Check sheet for the modelled part. Datum: model origin and axes. Units: mm. Round coordinates to 2 decimals unless told otherwise and drop trailing zeros. Loops run counter-clockwise (first coordinate to the right, second up) from the corner with the lowest first, then second, coordinate; pieces in that order, holes last. Notation, with made-up numbers: (43, 71.5) -> (95, 71.5) arc R23 ccw to (95, 81.5) -> close; hole circle Ø3 at (-6.75, 19.5). An arc over 180 degrees is marked (long way). One line per question, with ' | ' between items.
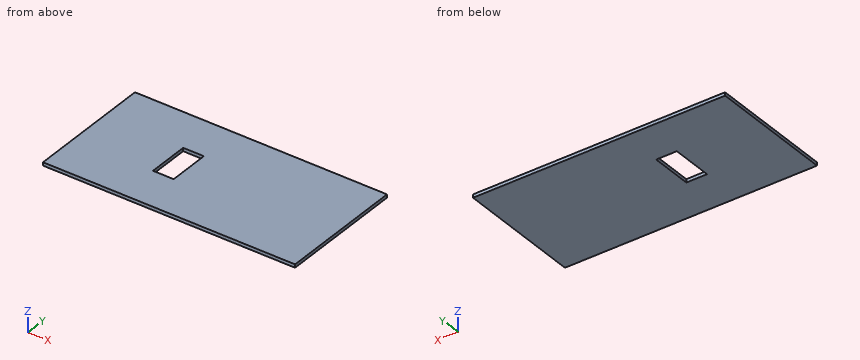
Autodesk Inventor part; units mm, degrees
ref_plane "YZ Plane" through (0, 0, 0) normal (1, 0, 0) x (0, 1, 0)
ref_plane "XZ Plane" through (0, 0, 0) normal (0, 1, 0) x (-1, 0, 0)
ref_plane "XY Plane" through (0, 0, 0) normal (0, 0, 1) x (1, 0, 0)
sketch "Sketch1" plane through (0, 0, 0) normal (0, 0, 1) x (1, 0, 0)
  line L0 (0, 0) -> (1219.2, 0)
  line L1 (1219.2, 0) -> (1219.2, 609.6)
  line L2 (1219.2, 609.6) -> (0, 609.6)
  line L3 (0, 609.6) -> (0, 0)
  dimension "d0" = 1219.2
  dimension "d1" = 609.6
extrude "Extrusion1" add sketch "Sketch1" along normal blind 15.875
sketch "Sketch6" plane through (0, 0, 15.875) normal (0, 0, 1) x (1, 0, 0)
  line L0 (482.6, 404.8) -> (382.6, 404.8)
  line L1 (482.6, 204.8) -> (382.6, 204.8)
  line L2 (382.6, 204.8) -> (382.6, 404.8)
  line L3 (482.6, 404.8) -> (482.6, 204.8)
extrude "Extrusion5" cut sketch "Sketch6" against normal blind 90
properties part number "Window Gyp Board"
(1) Sectioned sample at B-B, the plane z = 7.5. Record the cut outline in (x, y).
Answer:
outline: (0, 0) -> (1219.2, 0) -> (1219.2, 609.6) -> (0, 609.6) -> close; hole (382.6, 204.8) -> (482.6, 204.8) -> (482.6, 404.8) -> (382.6, 404.8) -> close
(2) Scan lines: probe 1 along X at (y, z) = (241, 3); probe 2 along Y at (x, z) = (442, 2). Record each from-to range of solid material in increasing order.
Answer:
probe 1: x = 0 to 382.6, 482.6 to 1219.2 | probe 2: y = 0 to 204.8, 404.8 to 609.6
(3) Sectioned sample at A-A, the plane y = 229. Record the cut outline in (x, z) (3 decimals), and give its area (3 significant figures).
Answer:
outline: (0, 0) -> (382.6, 0) -> (382.6, 15.875) -> (0, 15.875) -> close; (482.6, 0) -> (1219.2, 0) -> (1219.2, 15.875) -> (482.6, 15.875) -> close | area: 17,800 mm2
